from build123d import *

# Parameters (mm, degrees)
F0_R      = 30
F1_DEPTH  = 20
F3_DEPTH  = 10
F5_DEPTH  = 25
F7_DEPTH  = 10
F9_DEPTH  = 5
F10_R     = 20
F11_DEPTH = 20


with BuildPart() as f1:
    # F0 (on Top) → F1 (new body)
    with BuildSketch(Plane.XY):
        Circle(F0_R)
    extrude(amount=F1_DEPTH)

    # F2 (on Top) → F3 (join)
    with BuildSketch(Plane.XY):
        with BuildLine():
            ThreePointArc((22.36068, 20), (30, 0), (22.36068, -20))
            Line((22.36068, -20), (80, -20))
            Line((80, -20), (80, 20))
            Line((80, 20), (22.36068, 20))
        make_face()
        with BuildLine():
            Line((20, -80), (20, -22.36068))
            ThreePointArc((20, -22.36068), (0, -30), (-20, -22.36068))
            Line((-20, -22.36068), (-20, -80))
            Line((-20, -80), (20, -80))
        make_face()
    extrude(amount=F3_DEPTH)

    # F4 (on face) → F5 (cut)
    with BuildSketch(Plane.XY.offset(10)):
        with BuildLine():
            Line((7.5, -80), (7.5, -50))
            ThreePointArc((7.5, -50), (0, -42.5), (-7.5, -50))
            Line((-7.5, -50), (-7.5, -80))
            Line((-7.5, -80), (7.5, -80))
        make_face()
    extrude(amount=-F5_DEPTH, mode=Mode.SUBTRACT)

    # F6 (on face) → F7 (cut)
    with BuildSketch(Plane.XY.offset(10)):
        with BuildLine():
            Line((80, 7.5), (50, 7.5))
            ThreePointArc((50, 7.5), (42.5, 0), (50, -7.5))
            Line((50, -7.5), (80, -7.5))
            Line((80, -7.5), (80, 7.5))
        make_face()
    extrude(amount=-F7_DEPTH, mode=Mode.SUBTRACT)

    # F8 (on Top) → F9 (cut)
    with BuildSketch(Plane.XY):
        with BuildLine():
            ThreePointArc((20, -34.641016), (0, -40), (-20, -34.641016))
            Line((-20, -34.641016), (-20, -80))
            Line((-20, -80), (20, -80))
            Line((20, -80), (20, -34.641016))
        make_face()
        with BuildLine():
            ThreePointArc((34.641016, 20), (40, 0), (34.641016, -20))
            Line((34.641016, -20), (80, -20))
            Line((80, -20), (80, 20))
            Line((80, 20), (34.641016, 20))
        make_face()
    extrude(amount=F9_DEPTH, mode=Mode.SUBTRACT)

    # F10 (on face) → F11 (cut)
    with BuildSketch(Plane.XY.offset(20)):
        Circle(F10_R)
    extrude(amount=-F11_DEPTH, mode=Mode.SUBTRACT)


solid = f1.part
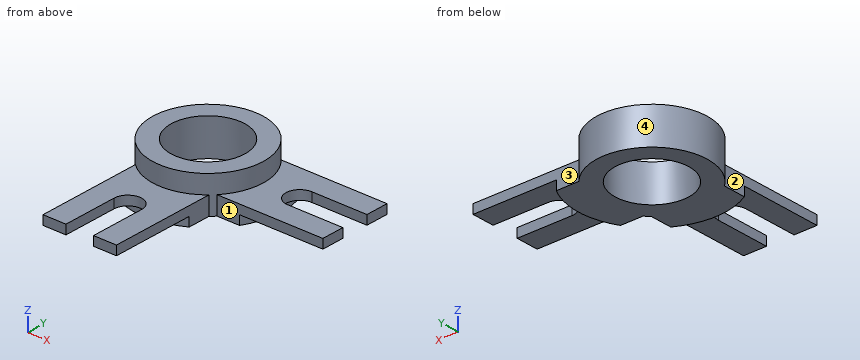
The listing builds one solid part. Answer for the finished solid, in the listing's coordinates (mm). Face numbers are marked on the shaded views. A direction names the side the tool comes from. Round coordinates to 2 decimals unless told otherwise and drop trailing zeros. Loops run counter-clockwise (first coordinate to the right, second up) from the corner with the lowest first, then second, coordinate; pieces in that order, holes last. Notation, with made-up numbers: M -37,-28.5 L -31,-28.5 A32 cw -31,4.5 Z; hole C 62,-35.75 d5. An arc over 180 degrees is marked long. Write each question's results on one line, items separated by ' | '. Start each with the question number.
1) Each of these flat-tipped pins is pushed along its axis until it touches: pin 1 (2 mm diameter, centred on x = -0.5, z = 4.5, fed in from +Y); pin 2 (5.5 mm diameter, centred on y = -70, z = 7.5, fed in from +X); pin 3 (5 mm diameter, centred on y = -58, z = 5, fed in from -X); pin 4 (11 mm diameter, centred on x = 54.5, z = 2.5, fed in from -Y). Where does it stop, or does it pass through?
2) Find section B-B on y = 0. Write down the section's boundary in (x, z).
3) Find section C-C on z = 1.75. Write down the section's boundary in (x, y), plus the area to 3 significant figures.
4) Straight lines are drawn through the part: probe 1 along Y at (x, z) = (57.5, 8.75); probe 2 along Y at (x, z) = (0, 7.5); probe 3 along X at (y, z) = (-23.5, 4). For each, find the intervals that lie inside material, in ascending order.
5) Find section A-A on x = 0. Write down the section's boundary in (y, z).
6) Find section D-D on y = -64. Write down the section's boundary in (x, z).
7) Which of the six approach directions +Z, -Z, +X, -X, +Y, -Y give full straight-line access (tool end or side, diameter ignored) to the marked faces 1, 2, 3 and 4?
Final values:
1) pin 1: y = 30 | pin 2: x = 20 | pin 3: x = -20 | pin 4: y = -20
2) outline: M -30,0 L -20,0 L -20,20 L -30,20 Z; M 20,0 L 40,0 L 40,5 L 42.5,5 L 42.5,10 L 30,10 L 30,20 L 20,20 Z
3) outline: M -20,-34.64 A40 ccw 20,-34.64 L 20,-22.36 A30 ccw 22.36,-20 L 34.64,-20 A40 ccw 34.64,20 L 22.36,20 A30 ccw long -20,-22.36 Z; hole C 0,0 d40 | area: 2,420 mm²
4) probe 1: -20 to -7.5, 7.5 to 20 | probe 2: -42.5 to -20, 20 to 30 | probe 3: -20 to 20
5) outline: M -42.5,5 L -40,5 L -40,0 L -20,0 L -20,20 L -30,20 L -30,10 L -42.5,10 Z; M 20,0 L 30,0 L 30,20 L 20,20 Z
6) outline: M -20,5 L -7.5,5 L -7.5,10 L -20,10 Z; M 7.5,5 L 20,5 L 20,10 L 7.5,10 Z
7) face 1: +Z, -Z, +X, -Y | face 2: +Z, -Z, -X, -Y | face 3: +Z, -Z, +X, +Y | face 4: +Z
